from build123d import *

# Parameters (mm, degrees)
F0_R     = 3.175
F1_DEPTH = 25.4


with BuildPart() as f1:
    # F0 (on Front) → F1 (new body)
    with BuildSketch(Plane.XZ):
        Polygon((94.2848, 0), (0, 0), (0, -25.4), (25.4508, -25.4), (25.4508, -9.525), (61.2648, -9.525), (61.2648, -25.4), (94.2848, -25.4), align=None)
        with Locations((15.875, -9.525)):
            Circle(F0_R, mode=Mode.SUBTRACT)
        with Locations((78.486, -9.525)):
            Circle(F0_R, mode=Mode.SUBTRACT)
    extrude(amount=F1_DEPTH)


solid = f1.part
The listing builds one solid part. Answer for the finished solid, in the listing's coordinates (mm). A direction names the side the tool comes from. Coordinates: 2 decimals unless noted, no trailing zeros. Write each loop counter-clockwise with the first axis right and the second up, starting at its lowest first coordinate (ties: lowest second). Pieces come first, ordered by that corner, then holes. Notation, with made-up numbers: M 89.25,83 L 132.25,83 A8 ccw 132.25,88 Z; hole C 49,68.5 d9. An arc over 180 degrees is marked long. Write each question's results on one line, items separated by ' | '.
Item 1: Consider probe 1 along X at (y, z) = (-21, -11.75); probe 2 along X at (y, z) = (-21.25, -18.5); probe 3 along Z at (x, y) = (37, -20.75) (3 decimals). Determine where each line is inside the solid, lowest interval first. Write a range as [from, to].
Answer below:
probe 1: [0, 13.61], [18.14, 25.45], [61.26, 76.22], [80.75, 94.28] | probe 2: [0, 25.45], [61.26, 94.28] | probe 3: [-9.525, 0]
Item 2: Which of the six approach directions +Z, -Z, +X, -X, +Y, -Y give full straight-line access (tool end or side, diameter ignored) to faces 4 (the face through (81.514, -12.522, -8.571)), 5 (the face through (43, -13, -9.525))?
Answer below:
face 4: +Y, -Y | face 5: -Z, +Y, -Y
Item 3: The part is cut by section D-D on x = 42. Determine the outline of the cut face in (y, z) (3 decimals), and give its area (3 significant figures).
Answer below:
outline: M -25.4,-9.525 L 0,-9.525 L 0,0 L -25.4,0 Z | area: 242 mm2
Item 4: The part is cut by section C-C on x = 17. Determine the outline of the cut face in (y, z), and give its area (3 significant figures).
Answer below:
outline: M -25.4,-25.4 L 0,-25.4 L 0,-12.49 L -25.4,-12.49 Z; M -25.4,-6.56 L 0,-6.56 L 0,0 L -25.4,0 Z | area: 494 mm2
Item 5: The part is cut by section B-B on z = -16.5. Determine the outline of the cut face in (x, y).
Answer below:
outline: M 0,-25.4 L 25.45,-25.4 L 25.45,0 L 0,0 Z; M 61.26,-25.4 L 94.28,-25.4 L 94.28,0 L 61.26,0 Z
Item 6: The part is cut by section A-A on y = -21.25. Determine the outline of the cut face in (x, z) (3 decimals).
Answer below:
outline: M 0,-25.4 L 25.451,-25.4 L 25.451,-9.525 L 61.265,-9.525 L 61.265,-25.4 L 94.285,-25.4 L 94.285,0 L 0,0 Z; hole C 15.875,-9.525 d6.35; hole C 78.486,-9.525 d6.35
Item 7: Given P1, Ø12.5, axis at x = 42, y = -14.5, coming from the -Z side (3 decimals); P2, Ø5, axis at x = 78.486, z = -9.525, coming from the -Y side, each flat-ended and moving along its own axis, determine where each tip first touches the part or whether it passes through.
Answer below:
P1: z = -9.525 | P2: through
Item 8: For a pull along X with two mould halves and no side action, classify faces 1 (the face through (94.285, -13, -13)), 2 (the face through (61.265, -13, -17)), 3 (the face through (78, -13, -25.4)) as released by +X, released by -X, zero draft, split by the parting line, or undercut.
Answer below:
face 1: released by +X | face 2: undercut | face 3: zero draft
